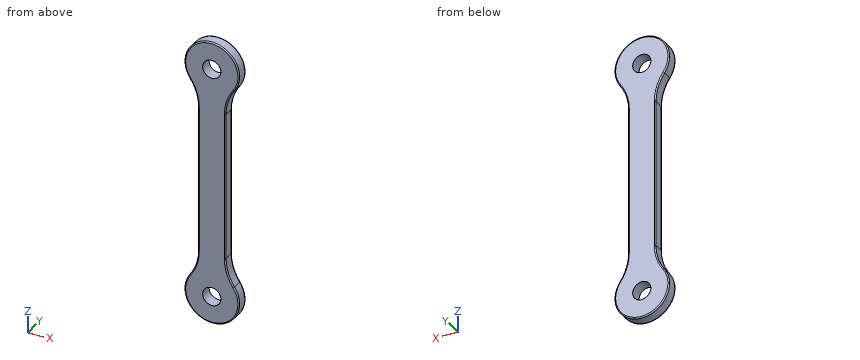
```python
from build123d import *

# Parameters (mm, degrees)
SKETCH1_R           = 2
BOSS_EXTRUDE1_DEPTH = 2.5
FILLET1_R           = 10
FILLET2_R           = 0.25


with BuildPart() as part:
    # Sketch1 → Boss-Extrude1 (new body)
    with BuildSketch(Plane(origin=(0, 0, 0), x_dir=(1, 0, 0), z_dir=(0, 1, 0))):
        with BuildLine():
            ThreePointArc((-3, -20.303847577), (0, -31.5), (3, -20.303847577))
            Line((3, -20.303847577), (3, 20.303847577))
            ThreePointArc((3, 20.303847577), (0, 31.5), (-3, 20.303847577))
            Line((-3, 20.303847577), (-3, -20.303847577))
        make_face()
        with Locations((0, -25.5)):
            Circle(SKETCH1_R, mode=Mode.SUBTRACT)
        with Locations((0, 25.5)):
            Circle(SKETCH1_R, mode=Mode.SUBTRACT)
    extrude(amount=BOSS_EXTRUDE1_DEPTH)

    # Fillet1
    fillet1_edges = [part.edges().sort_by_distance(p)[0] for p in [
        (-3, 1.25, 20.303847577),
        (-3, 1.25, -20.303847577),
        (3, 1.25, -20.303847577),
        (3, 1.25, 20.303847577),
    ]]
    fillet(fillet1_edges, radius=FILLET1_R)

    # Fillet2
    fillet2_edges = [part.edges().sort_by_distance(p)[0] for p in [
        (0, 0, 31.5),
        (0, 2.5, 31.5),
        (-3, 0, 0),
        (-3, 2.5, 0),
        (0, 0, -31.5),
        (0, 2.5, -31.5),
        (3, 0, 0),
        (3, 2.5, 0),
        (-3.480283618, 0, 19.234483125),
        (-3.480283618, 2.5, 19.234483125),
        (-3.480283618, 0, -19.234483125),
        (-3.480283618, 2.5, -19.234483125),
        (3.480283618, 0, -19.234483125),
        (3.480283618, 2.5, -19.234483125),
        (3.480283618, 0, 19.234483125),
        (3.480283618, 2.5, 19.234483125),
    ]]
    fillet(fillet2_edges, radius=FILLET2_R)


solid = part.part
```
The listing builds one solid part. Answer for the finished solid, in the listing's coordinates (mm). Give positions to 0.01 mm unless a question says otherwise; leave off trailing zeros. Order: outer loops, then holes, each group sorted by start corner. A loop starts at its lowest first (then second) coordinate and runs counter-clockwise, first axis right, second up. Notation, with made-up numbers: (50, -12) -> (96, -12) arc R27 ccw to (96, 10) -> close; hole circle Ø5 at (31, 77). An arc over 180 degrees is marked (long way). Answer as CSV lines item,"result". Start each with the question number.
Q1. A cutting plane is placed at C-C (z = 8). Determine the outline of the cut face in (x, y), then the cut area to 3 significant figures.
Q2. A cutting plane is placed at A-A (y = 1.75). Determine the outline of the cut face in (x, z) (3 decimals).
Q3. Given pin 1 (3 mm diameter, centred on x = 0, z = -25.5, fed in from +Y); pin 2 (1 mm diameter, centred on y = 1.5, z = 4.5, fed in from +X); pin 3 (1 mm diameter, centred on y = 1, z = 1, fed in from -X), each flat-ended and moving along its own axis, determine where each tip first touches the part or whether it passes through.
Q4. A cutting plane is placed at B-B (x = 0). Determine the outline of the cut face in (y, z).
Q5. Find the intervals of material crossed by L1, parallel to Z at x = 0, y = 0.9; L2, parallel to Z at x = -0.5, y = 1.7; L3, parallel to X at y = 0.6, z = -25.5, in increasing order.
Results found:
1,outline,"(-3, 0.25) arc R0.25 ccw to (-2.75, 0) -> (2.75, 0) arc R0.25 ccw to (3, 0.25) -> (3, 2.25) arc R0.25 ccw to (2.75, 2.5) -> (-2.75, 2.5) arc R0.25 ccw to (-3, 2.25) -> close"
1,area,"14.9 mm2"
2,outline,"(-4.875, -22.002) arc R6 ccw (long way) to (4.875, -22.002) arc R10 cw to (3, -16.173) -> (3, 16.173) arc R10 cw to (4.875, 22.002) arc R6 ccw (long way) to (-4.875, 22.002) arc R10 cw to (-3, 16.173) -> (-3, -16.173) arc R10 cw to start; hole circle Ø4 at (0, -25.5); hole circle Ø4 at (0, 25.5)"
3,pin 1,"through"
3,pin 2,"x = 3"
3,pin 3,"x = -3"
4,outline,"(0, -31.25) arc R0.25 ccw to (0.25, -31.5) -> (2.25, -31.5) arc R0.25 ccw to (2.5, -31.25) -> (2.5, -27.5) -> (0, -27.5) -> close; (0, -23.5) -> (2.5, -23.5) -> (2.5, 23.5) -> (0, 23.5) -> close; (0, 27.5) -> (2.5, 27.5) -> (2.5, 31.25) arc R0.25 ccw to (2.25, 31.5) -> (0.25, 31.5) arc R0.25 ccw to (0, 31.25) -> close"
5,L1,"-31.5 to -27.5, -23.5 to 23.5, 27.5 to 31.5"
5,L2,"-31.48 to -27.44, -23.56 to 23.56, 27.44 to 31.48"
5,L3,"-6 to -2, 2 to 6"
